from build123d import *

# Parameters (mm, degrees)
F1_DEPTH = 101.6
F2_DEPTH = 7.62
F3_R     = 5.08


with BuildPart() as f1:
    # F0 (on Top) → F1 (new body)
    with BuildSketch(Plane.XY):
        Polygon((33.728803, 58.42), (0, 58.42), (-33.728803, 58.42), (-67.457605, 0), (-33.728803, -58.42), (33.728803, -58.42), (67.457605, 0), align=None)
        Polygon((-58.658787, 0), (-29.329394, 50.8), (0, 50.8), (29.329394, 50.8), (58.658787, 0), (29.329394, -50.8), (-29.329394, -50.8), align=None, mode=Mode.SUBTRACT)
    extrude(amount=F1_DEPTH)

    # F0 (on Top) → F2 (join)
    with BuildSketch(Plane.XY):
        Polygon((0, 50.8), (-29.329394, 50.8), (-58.658787, 0), (-29.329394, -50.8), (29.329394, -50.8), (58.658787, 0), (29.329394, 50.8), align=None)
    extrude(amount=F2_DEPTH)

    # F3
    f3_edges = [f1.edges().sort_by_distance(p)[0] for p in [
        (33.728803, 58.42, 50.8),
        (0, 58.42, 101.6),
        (-33.728803, 58.42, 50.8),
        (0, 58.42, 0),
        (-67.457605, 0, 50.8),
        (-50.593204, 29.21, 0),
        (-50.593204, 29.21, 101.6),
        (-33.728803, -58.42, 50.8),
        (-50.593204, -29.21, 0),
        (-50.593204, -29.21, 101.6),
        (33.728803, -58.42, 50.8),
        (0, -58.42, 0),
        (0, -58.42, 101.6),
        (67.457605, 0, 50.8),
        (50.593204, 29.21, 0),
        (50.593204, 29.21, 101.6),
        (50.593204, -29.21, 0),
        (50.593204, -29.21, 101.6),
    ]]
    fillet(f3_edges, radius=F3_R)


solid = f1.part
Build history of the part. All positions in model axes, mm. A direction names the side the tool comes from. Give positions to 0.01 mm unless a question says otherwise; leave off trailing zeros. Write each loop counter-clockwise with the first axis right and the second up, starting at its lowest first coordinate (ties: lowest second). Pieces come first, ordered by that corner, then holes. Notation, with made-up numbers: (70, 80) - (126, 80) arc R26 cw to (126, 94) - close; hole circle Ø11 at (36.5, -39). An arc over 180 degrees is marked (long way). Use one line per item in the form item = value. Start each with the question number.
1. Probe line 1 (Y direction, x = 16.5, z = 88); line 2 (Y direction, x = 47, z = 84); line 3 (X direction, y = 9, z = 80.5). List the from-to ranges inside material, lowest first. Write a range as [from, to].
2. Band-saw the part on B-B on x = 12. Write the cut outline in (y, z).
3. 3-axis set-ups, long thin cutter, end or side, ignore diameter. For faces 4 (the face through (43.789, 25.756, 53.952)), 5 (the face through (-33.4, -57.7, 51.4)): which of +Z, -Z, +X, -X, +Y, -Y reach the whole face in a straight line?
4. Drop flat-ended pins along their axis: pin 1 Ø5 at (y, z) = (16.5, 24) entering from -X; pin 2 Ø1 at (y, z) = (-45, 76.5) entering from +X; pin 3 Ø5 at (x, z) = (-41.5, 69.5) entering from -Y; pin 4 Ø12 at (x, y) = (-53.5, 24) entering from +Z. Give the stop position or say it passes through.
5. Two-plate mould, pull along X, no slides. Class faces 1 (the face through (50.809, 28.837, 50.16)), 2 (the face through (-50.38, 29.58, 50.16)), 3 (the face through (-43.789, -25.756, 53.952)): released by +X, released by -X, zero draft, split by the parting line, or undercut.
6. Band-saw the part on A-A on z = 77. Write the cut outline in (x, y).
Conclusion:
q1.line_1 = [-58.42, -50.8], [50.8, 58.42]
q1.line_2 = [-35.43, -20.19], [20.19, 35.43]
q1.line_3 = [-62.26, -53.46], [53.46, 62.26]
q2.outline = (-58.42, 5.08) arc R5.08 ccw to (-53.34, 0) - (53.34, 0) arc R5.08 ccw to (58.42, 5.08) - (58.42, 96.52) arc R5.08 ccw to (53.34, 101.6) - (50.8, 101.6) - (50.8, 7.62) - (-50.8, 7.62) - (-50.8, 101.6) - (-53.34, 101.6) arc R5.08 ccw to (-58.42, 96.52) - close
q3.face_4 = +Z
q3.face_5 = +Z, -Z, -X, -Y
q4.pin_1 = -59.37
q4.pin_2 = 41.77
q4.pin_3 = -49.29
q4.pin_4 = 101.6
q5.face_1 = released by +X
q5.face_2 = released by -X
q5.face_3 = undercut
q6.outline = (-65.99, -2.54) - (-35.2, -55.88) arc R5.08 ccw to (-30.8, -58.42) - (30.8, -58.42) arc R5.08 ccw to (35.2, -55.88) - (65.99, -2.54) arc R5.08 ccw to (65.99, 2.54) - (35.2, 55.88) arc R5.08 ccw to (30.8, 58.42) - (-30.8, 58.42) arc R5.08 ccw to (-35.2, 55.88) - (-65.99, 2.54) arc R5.08 ccw to start; hole (-58.66, 0) - (-29.33, -50.8) - (29.33, -50.8) - (58.66, 0) - (29.33, 50.8) - (-29.33, 50.8) - close
